Here's how the part is built. I have some questions about the finished solid (model axes, mm). A direction names the side the tool comes from. Coordinates: 2 decimals unless noted, no trailing zeros. Order: outer loops, then holes, each group sorted by start corner. A loop starts at its lowest first (then second) coordinate and runs counter-clockwise, first axis right, second up. Notation, with made-up numbers: (75.25, 77.5) - (133.25, 77.5) arc R14 ccw to (133.25, 101.5) - close; hole circle Ø1 at (37, -38). An arc over 180 degrees is marked (long way). Answer as CSV lines item,"result". Start each with the question number.
Item 1: We'd pull the mould along Y, two halves only. Please class faces 1 (the face through (16, 0, -8)), 2 (the face through (-9.94, 67.38, -9.67)), 3 (the face through (16, 45, 0)): pulls with the +Y half, pulls with the -Y half, needs draft (parallel to the pull), parting line crosses it, or undercut.
Item 2: On a 3-axis mill with a long thin cutter (end or side, diameter ignored), from which of +Z, -Z, +X, -X, +Y, -Y can I reach the whole of each face in a straight line? I mean faces 4 (the face through (29, 45, -6.35)), 5 (the face through (16, -20, -8)), 6 (the face through (0, -26, -3)), 7 (the face through (16, -26.35, -16)). Say none if no direction works.
Item 3: Imagine slicing it at C-C on x = 23.5. List the corners of the cut face in (y, z) for me.
Item 4: Imagine slicing it at D-D on z = -10. List the corners of the cut face in (x, y) for me, and give its area (3 significant figures).
Item 5: I'm going to push flat-ended pins straight in: pin 1 (5 mm diameter, centred on y = 37.5, z = -19, fed in from -X); pin 2 (1 mm diameter, centred on x = 14.5, y = -18.5, fed in from +Z); pin 3 (5 mm diameter, centred on y = 25, z = -2.5, fed in from -X); pin 4 (3 mm diameter, centred on x = -8, y = 74, fed in from +Z). Where does each tip first touch, or does it pass through?
Item 6: Imagine slicing it at B-B on y = 50.5. List the corners of the cut face in (x, z) for me, and give its area (3 significant figures).
Item 7: Imagine slicing it at A-A on z = -3. List the corners of the cut face in (x, y) for me.
Item 8: I need wall thicknesses on line 1 (Y direction, x = 13.5, z = -9.25); line 2 (X direction, y = 4.5, z = -10.5); line 3 (Y direction, x = 15, z = -4.75). Which ranges of each line are inside material? Lowest first, please.
from build123d import *

# Parameters (mm, degrees)
BOSS_EXTRUDE1_DEPTH = 32.7
SKETCH3_W           = 6.35
SKETCH3_H           = 20
CUT_EXTRUDE2_DEPTH  = 129.269452716
SKETCH7_R           = 2.5
BOSS_EXTRUDE4_DEPTH = 33.05


with BuildPart() as part:
    # Sketch2 → Boss-Extrude1 (new body)
    with BuildSketch(Plane(origin=(0, 0, 0), x_dir=(0, 0, -1), z_dir=(1, 0, 0))):
        Polygon((0, 0), (20, 0), (20, -20), (0, -20), (0, -32.7), (6.35, -32.7), (6.35, -26.35), (26.35, -26.35), (26.35, 88.5), (0, 88.5), align=None)
    extrude(amount=BOSS_EXTRUDE1_DEPTH)

    # Sketch3 → Cut-Extrude2 (cut, through all)
    with BuildSketch(Plane(origin=(0, 88.5, 0), x_dir=(1, 0, 0), z_dir=(0, 1, 0))):
        with Locations((3.175, 16.35)):
            Rectangle(SKETCH3_W, SKETCH3_H)
        with Locations((29.525, 16.35)):
            Rectangle(SKETCH3_W, SKETCH3_H)
    extrude(amount=-CUT_EXTRUDE2_DEPTH, mode=Mode.SUBTRACT)

    # Sketch7 → Boss-Extrude4 (add)
    with BuildSketch(Plane.ZY.offset(-6.35)):
        with Locations(Location((-10, 69.86, 0), (0, 0, 180))):
            Circle(SKETCH7_R)
    extrude(amount=BOSS_EXTRUDE4_DEPTH)


solid = part.part
Responses:
1,face 1,"undercut"
1,face 2,"parting line crosses it"
1,face 3,"needs draft"
2,face 4,"-Z, +X, +Y, -Y"
2,face 5,"+Z, +X, -X"
2,face 6,"+Z, -Z, -X, +Y, -Y"
2,face 7,"-Z, +X, -X, -Y"
3,outline,"(-32.7, -6.35) - (-26.35, -6.35) - (-26.35, -26.35) - (88.5, -26.35) - (88.5, 0) - (0, 0) - (0, -20) - (-20, -20) - (-20, 0) - (-32.7, 0) - close"
4,outline,"(-26.7, 67.36) - (6.35, 67.36) - (6.35, 0) - (26.35, 0) - (26.35, 88.5) - (6.35, 88.5) - (6.35, 72.36) - (-26.7, 72.36) - close; (6.35, -26.35) - (26.35, -26.35) - (26.35, -20) - (6.35, -20) - close"
4,area,"2,060 mm^2"
5,pin 1,"stops at x = 6.35"
5,pin 2,"stops at z = -20"
5,pin 3,"stops at x = 0"
5,pin 4,"passes through"
6,outline,"(0, -6.35) - (6.35, -6.35) - (6.35, -26.35) - (26.35, -26.35) - (26.35, -6.35) - (32.7, -6.35) - (32.7, 0) - (0, 0) - close"
6,area,"608 mm^2"
7,outline,"(0, -32.7) - (32.7, -32.7) - (32.7, -20) - (0, -20) - close; (0, 0) - (32.7, 0) - (32.7, 88.5) - (0, 88.5) - close"
8,line 1,"y = -26.35 to -20, 0 to 88.5"
8,line 2,"x = 6.35 to 26.35"
8,line 3,"y = -32.7 to -20, 0 to 88.5"
